from build123d import *

# Parameters (mm, degrees)
F0_R     = 2.8575
F0_R_2   = 0.889
F0_R_3   = 1.905
F0_R_4   = 11.7475
F1_DEPTH = 4.318
F2_W     = 12.7
F2_H     = 4.318
F3_DEPTH = 3.175
F4_R     = 5.08
F6_DEPTH = 25.4
F7_R     = 5.08
F8_R     = 0.762


# Not quite as in the source:
# - a feature names something its author has since deleted; it is built from what else it names


with BuildPart() as f1:
    # F0 (on Top) → F1 (new body)
    with BuildSketch(Plane.XY):
        Polygon((0, -20.7006), (0, 0), (0, 63.5), (-41.91, 63.5), (-41.91, 19), (-41.91, 0), (-41.91, -20.7006), align=None)
        with Locations((-34.925, -12.09)):
            Circle(F0_R, mode=Mode.SUBTRACT)
        with Locations((-34.925, 9.5)):
            Circle(F0_R, mode=Mode.SUBTRACT)
        with Locations((-6.985, -12.09)):
            Circle(F0_R, mode=Mode.SUBTRACT)
        with Locations((-1.27, -4.47)):
            Circle(F0_R_2, mode=Mode.SUBTRACT)
        with Locations((-6.985, 9.5)):
            Circle(F0_R, mode=Mode.SUBTRACT)
        with Locations((-1.27, 1.88)):
            Circle(F0_R_2, mode=Mode.SUBTRACT)
        with Locations((-36.83, 27.178)):
            Circle(F0_R_3, mode=Mode.SUBTRACT)
        with Locations((-36.83, 58.293)):
            Circle(F0_R_3, mode=Mode.SUBTRACT)
        with Locations((-5.08, 27.178)):
            Circle(F0_R_3, mode=Mode.SUBTRACT)
        with Locations((-20.955, 42.7355)):
            Circle(F0_R_4, mode=Mode.SUBTRACT)
        with Locations((-5.08, 58.293)):
            Circle(F0_R_3, mode=Mode.SUBTRACT)
    extrude(amount=F1_DEPTH)

    # F2 (on face) → F3 (join)
    with BuildSketch(Plane.YZ):
        with Locations((-1.2696, 2.159)):
            Rectangle(F2_W, F2_H)
    extrude(amount=F3_DEPTH)

    # F4
    f4_edges = [f1.edges().sort_by_distance(p)[0] for p in [
        (0, 63.5, 2.159),
        (-41.91, 63.5, 2.159),
        (0, -20.7006, 2.159),
        (-41.91, -20.7006, 2.159),
    ]]
    fillet(f4_edges, radius=F4_R)

    # F5 (on face) → F6 (cut)
    with BuildSketch(Plane.XY.offset(4.318)):
        Polygon((-51.067360534, -23.478101939), (-14.478, -25.962697342), (-14.478, 18.2829182773), (4.9410860353, 18.2829182773), (4.9410860353, 69.2363290038), (-51.067360534, 69.2363290038), align=None)
    extrude(amount=-F6_DEPTH, mode=Mode.SUBTRACT)

    # F7
    f7_edges = [f1.edges().sort_by_distance(p)[0] for p in [
        (-14.478, -20.7006, 2.159),
        (-14.478, 18.282918, 2.159),
        (0, 18.282918, 2.159),
    ]]
    fillet(f7_edges, radius=F7_R)

    # F8
    f8_edges = [f1.edges().sort_by_distance(p)[0] for p in [
        (0, 9.141659, 4.318),
        (-1.487898, 16.795021, 4.318),
        (1.5875, 5.0804, 4.318),
        (-7.239, 18.282918, 4.318),
        (3.175, -1.2696, 4.318),
        (-12.990102, 16.795021, 4.318),
        (1.5875, -7.6196, 4.318),
        (-14.478, -1.208841, 4.318),
        (0, -11.6201, 4.318),
        (-12.990102, -19.212702, 4.318),
        (-1.487898, -19.212702, 4.318),
        (-7.239, -20.7006, 4.318),
        (-9.8425, -12.09, 4.318),
        (-2.159, -4.47, 4.318),
        (-2.159, 1.88, 4.318),
        (-9.8425, 9.5, 4.318),
    ]]
    fillet(f8_edges, radius=F8_R)


solid = f1.part
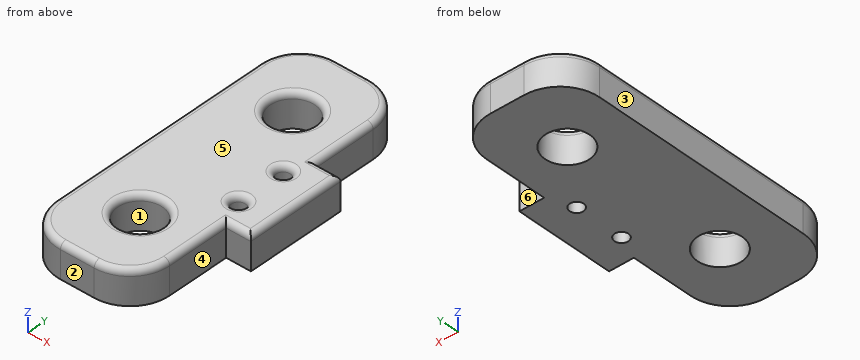
Here's how the part is built. I have some questions about the finished solid (model axes, mm). Face numbers are marked on the shaded views. A direction names the side the tool comes from. Give positions to 0.01 mm unless a question says otherwise; leave off trailing zeros. Order: outer loops, then holes, each group sorted by start corner. A loop starts at its lowest first (then second) coordinate and runs counter-clockwise, first axis right, second up. Notation, with made-up numbers: M -2,-27.75 L 24,-27.75 A21 cw 24,-11.75 Z; hole C 81.25,74.5 d3. An arc over 180 degrees is marked long. Answer as a JSON object with one key per item and string values. Group by question number.
1) Suppose I cut it at A-A, the plane y = -4.47. Write out the boundary of the cut face in (x, z) (3 decimals), plus the area to 4 significant figures.
2) Suppose I cut it at C-C, the plane y = 9.5. Write out the boundary of the cut face in (x, z).
3) On a 3-axis mill with a long thin cutter (end or side, diameter ignored), from which of +Z, -Z, +X, -X, +Y, -Y can I reach the whole of each face in a straight line? I mean the marked faces 4, 5 and 6. Say none if no direction works.
4) Please list where these lines run through material, in increasing order: L1, parallel to Y at x = -1.27, z = 2.1; L2, parallel to Y at x = -6.5, z = 1.8; L3, parallel to X at y = 2, z = 2.35 (3 decimals). Write a range as [from, to].
5) Suppose I cut it at D-D, the plane x = -6.75. Count the separate pieces of the cut face and the enclosed holes in it, plus the area to 3 significant figures.
6) Suppose I cut it at B-B, the plane z = 0.65. Write out the boundary of the cut face in (x, y) (1 decimal).
7) We'd pull the mould along Y, two halves only. Please class the marked faces 1, 2 and 3: pulls with the +Y half, pulls with the -Y half, needs draft (parallel to the pull), parting line crosses it, or undercut.
8) I'm going to push flat-ended pins straight in: pin 1 Ø4.5 at (x, y) = (-6.985, 9.5) entering from -Z; pin 2 Ø1.1 at (y, z) = (8.5, 1.5) entering from +X; pin 3 Ø1 at (x, z) = (2, 1) entering from -Y; pin 4 Ø1.6 at (x, z) = (1.5, 2) entering from +Y. Where does each tip first touch, or does it pass through?
Results found:
{
 "1": {"outline": "M -14.478,0 L -2.159,0 L -2.159,3.556 A0.762 ccw -2.921,4.318 L -13.716,4.318 A0.762 ccw -14.478,3.556 Z; M -0.381,0 L 3.175,0 L 3.175,3.556 A0.762 ccw 2.413,4.318 L 0.381,4.318 A0.762 ccw -0.381,3.556 Z", "area": "68.05 mm²"},
 "2": {"outline": "M -14.48,0 L -9.84,0 L -9.84,3.56 A0.76 ccw -10.6,4.32 L -13.72,4.32 A0.76 ccw -14.48,3.56 Z; M -4.13,0 L 0,0 L 0,3.56 A0.76 ccw -0.76,4.32 L -3.37,4.32 A0.76 ccw -4.13,3.56 Z"},
 "3": {"face 4": "+Z, -Z, +X, -Y", "face 5": "+Z, +X, -X, +Y, -Y", "face 6": "+Z, -Z, +X, +Y"},
 "4": {"L1": "[-18.98, -5.36], [-3.58, 0.99], [2.77, 16.56]", "L2": "[-20.7, -14.91], [-9.27, 6.68], [12.32, 18.28]", "L3": "[-14.478, -2.151], [-0.389, 3.175]"},
 "5": {"separate pieces": "3", "enclosed holes": "0", "area": "118 mm²"},
 "6": {"outline": "M -14.5,-15.6 A5.1 ccw -9.4,-20.7 L -5.1,-20.7 A5.1 ccw 0,-15.6 L 0,-7.6 L 3.2,-7.6 L 3.2,5.1 L 0,5.1 L 0,13.2 A5.1 ccw -5.1,18.3 L -9.4,18.3 A5.1 ccw -14.5,13.2 Z; hole C -7,-12.1 d5.7; hole C -7,9.5 d5.7; hole C -1.3,-4.5 d1.8; hole C -1.3,1.9 d1.8"},
 "7": {"face 1": "undercut", "face 2": "pulls with the -Y half", "face 3": "needs draft"},
 "8": {"pin 1": "through", "pin 2": "x = 0", "pin 3": "y = -7.62", "pin 4": "y = 5.08"}
}
